Autodesk Inventor part; units mm, degrees
ref_plane "YZ Plane" through (0, 0, 0) normal (1, 0, 0) x (0, 1, 0)
ref_plane "XZ Plane" through (0, 0, 0) normal (0, 1, 0) x (-1, 0, 0)
ref_plane "XY Plane" through (0, 0, 0) normal (0, 0, 1) x (1, 0, 0)
sketch "Sketch1" plane through (0, 0, 0) normal (0, 1, 0) x (-1, 0, 0)
  line L0 (-6.3436, 0) -> (7.6564, 0)
  line L1 (7.6564, 0) -> (7.6564, 10)
  line L2 (3.4064, 10) -> (3.4064, 2.5)
  line L3 (3.4064, 2.5) -> (-2.0936, 2.5)
  line L4 (-2.0936, 2.5) -> (-2.0936, 10)
  line L5 (-6.3436, 10) -> (-6.3436, 0)
  line L6 (-6.3436, 10) -> (-2.0936, 10)
  line L7 (3.4064, 10) -> (7.6564, 10)
  point P0 (0, 0)
  dimension "d0" = 10
  dimension "d2" = 14
  dimension "d3" = 2.5
  dimension "d24" = 4.25
  dimension "d25" = 4.25
extrude "Extrusion1" add sketch "Sketch1" along normal blind 6.1
sketch "Sketch2" plane through (6.3436, 0, 0) normal (0, 0, -1) x (-1, 0, 0)
  line L0 (0, 0) -> (0, 6.1)
  line L1 (2.25, 4.5071) -> (2.75, 4.5071)
  line L2 (2.75, 4.5071) -> (2.75, 4.0071)
  line L3 (2.75, 4.0071) -> (2.25, 4.0071)
  line L4 (2.25, 4.0071) -> (2.25, 4.5071)
  line L5 (2.25, 1.6957) -> (2.75, 1.6957)
  line L6 (2.75, 1.6957) -> (2.75, 1.1957)
  line L7 (2.75, 1.1957) -> (2.25, 1.1957)
  line L8 (2.25, 1.1957) -> (2.25, 1.6957)
  line L9 (11.75, 4.5071) -> (12.25, 4.5071)
  line L10 (12.25, 4.5071) -> (12.25, 4.0071)
  line L11 (11.75, 4.0071) -> (11.75, 4.5071)
  line L12 (12.25, 4.0071) -> (11.75, 4.0071)
  line L13 (11.75, 1.6957) -> (12.25, 1.6957)
  line L14 (12.25, 1.6957) -> (12.25, 1.1957)
  line L15 (11.75, 1.1957) -> (11.75, 1.6957)
  line L16 (12.25, 1.1957) -> (11.75, 1.1957)
  point P0 (6.3436, 0)
  dimension "d6" = 0.5
  dimension "d10" = 0.5
  dimension "d11" = 0.5
  dimension "d12" = 0.5
  dimension "d13" = 0.5
  dimension "d14" = 0.5
  dimension "d15" = 0.5
  dimension "d16" = 0.5
  dimension "d17" = 2.3114
  dimension "d18" = 9
  dimension "d19" = 2.25
extrude "Extrusion2" add sketch "Sketch2" along normal blind 3.8
properties part number "tacometer_ct" material "ABS Plastic"
Design review of the part built by this model. Coordinates are the model's own, in mm. A direction names the side the tool comes from. Coordinates: 2 decimals unless noted, no trailing zeros. Order: outer loops, then holes, each group sorted by start corner. A loop starts at its lowest first (then second) coordinate and runs counter-clockwise, first axis right, second up.
Item 1: For faces 1 (the flat face through (4, 3, 10)), 2 (the flat face through (-1, 3, 2.5)), list the 3-axis set-ups (+Z, -Z, +X, -X, +Y, -Y) from which the entire face can be reached by the end or side of a thin tool; tool diameter is ignored.
Item 2: For pin 1 Ø0.6 at (y, z) = (1.5, -2) entering from +X, flat-tipped, find the tip position at first contact; note if it passes through.
Item 3: Take a section at A-A, the plane z = 4. Write out the cut boundary in (x, y).
Item 4: Take a section at B-B, the plane z = -2.5. Write out the cut boundary in (x, y).
Item 5: Take a section at C-C, the plane y = 3.5. Write out the cut boundary in (x, z), then the cut area to 4 significant figures.
Item 6: Take a section at D-D, the plane x = 4.5. Write out the cut boundary in (y, z), then the cut area to 3 significant figures.
Item 7: The part is to be moulded in two halves that separate along X. For faces 3 (the flat face through (6.344, 3, 5)), 4 (the flat face through (2.094, 3, 6)), 5 (the flat face through (-6, 3, 10)), 6 (the flat face through (-3.406, 3, 6)), say which applies: pulls with the +X half, pulls with the -X half, needs draft (parallel to the pull), parting line crosses it, or undercut.
Item 8: For line 1 (Y direction, x = -5.5, z = -2); line 2 (X direction, y = 1.75, z = 7); line 3 (X direction, y = 1.5, z = -1.75), list the stretches that pass through material, from the lowest coordinate up.
The answers:
1. face 1: +Z, +X, -X, +Y, -Y
1. face 2: +Z, +Y, -Y
2. pin 1: stops at x = 4.09
3. outline: (-7.66, 0) - (-3.41, 0) - (-3.41, 6.1) - (-7.66, 6.1) - close; (2.09, 0) - (6.34, 0) - (6.34, 6.1) - (2.09, 6.1) - close
4. outline: (-5.91, 1.2) - (-5.41, 1.2) - (-5.41, 1.7) - (-5.91, 1.7) - close; (-5.91, 4.01) - (-5.41, 4.01) - (-5.41, 4.51) - (-5.91, 4.51) - close; (3.59, 1.2) - (4.09, 1.2) - (4.09, 1.7) - (3.59, 1.7) - close; (3.59, 4.01) - (4.09, 4.01) - (4.09, 4.51) - (3.59, 4.51) - close
5. outline: (-7.66, 0) - (6.34, 0) - (6.34, 10) - (2.09, 10) - (2.09, 2.5) - (-3.41, 2.5) - (-3.41, 10) - (-7.66, 10) - close
5. area: 98.75 mm2
6. outline: (0, 0) - (6.1, 0) - (6.1, 10) - (0, 10) - close
6. area: 61.0 mm2
7. face 3: pulls with the +X half
7. face 4: undercut
7. face 5: needs draft
7. face 6: undercut
8. line 1: y = 1.2 to 1.7, 4.01 to 4.51
8. line 2: x = -7.66 to -3.41, 2.09 to 6.34
8. line 3: x = -5.91 to -5.41, 3.59 to 4.09
